Check sheet for the modelled part. Datum: model origin and axes. Units: mm. Round coordinates to 2 decimals unless told otherwise and drop trailing zeros. Write item = value, one per line.
from build123d import *

# Parameters (mm, degrees)
SKETCH1_W                                          = 308.737
SKETCH1_H                                          = 580.9742
BOSS_EXTRUDE1_STOCK_DEPTH                          = 6.35
CUT_EXTRUDE1_MOUNTING_DEPTH                        = 658.943674439
CUT_EXTRUDE1_MOUNTING_DEPTH_BACK                   = 658.943674439
SKETCH2_R                                          = 3.175
CUT_EXTRUDE2_ELEVATOR_CLEARANCE_DEPTH              = 658.943674439
CUT_EXTRUDE2_ELEVATOR_CLEARANCE_DEPTH_BACK         = 658.943674439
SKETCH3_W                                          = 66.04
SKETCH3_H                                          = 431.1142
CUT_EXTRUDE3_SCORER_ANGLE_MATERIAL_REMO_DEPTH      = 658.943674439
CUT_EXTRUDE3_SCORER_ANGLE_MATERIAL_REMO_DEPTH_BACK = 658.943674439
CUT_EXTRUDE4_ALGAE_BEARING_HOLES_DEPTH             = 658.943674439
CUT_EXTRUDE4_ALGAE_BEARING_HOLES_DEPTH_BACK        = 658.943674439
SKETCH5_R                                          = 14.224
CUT_EXTRUDE5_MOTOR_MOUNTING_HOLES_DEPTH            = 658.943674439
CUT_EXTRUDE5_MOTOR_MOUNTING_HOLES_DEPTH_BACK       = 658.943674439
SKETCH6_R                                          = 2.5527
CUT_EXTRUDE6_ALGAE_FITMENT_DEPTH                   = 658.943674439
CUT_EXTRUDE6_ALGAE_FITMENT_DEPTH_BACK              = 658.943674439
SKETCH7_R                                          = 203.2
CUT_EXTRUDE7_TOP_BOTTOM_MOUNTING_DEPTH             = 658.943674439
CUT_EXTRUDE7_TOP_BOTTOM_MOUNTING_DEPTH_BACK        = 658.943674439
SKETCH8_R                                          = 2.5527
FILLET1_R                                          = 101.6
FILLET2_R                                          = 101.6
FILLET3_R                                          = 12.7
CUT_EXTRUDE1_DEPTH                                 = 658.943674439
CUT_EXTRUDE1_DEPTH_BACK                            = 658.943674439
SKETCH9_R                                          = 3.175
CUT_EXTRUDE2_DEPTH                                 = 658.943674439
CUT_EXTRUDE2_DEPTH_BACK                            = 658.943674439
SKETCH11_R                                         = 2.5527
CUT_EXTRUDE3_DEPTH                                 = 658.943674439
CUT_EXTRUDE3_DEPTH_BACK                            = 658.943674439
SKETCH12_R                                         = 2.5527


with BuildPart() as part:
    # Sketch1 → Boss-Extrude1 _Stock (new body)
    with BuildSketch(Plane.XY):
        with Locations((154.3685, 290.4871)):
            Rectangle(SKETCH1_W, SKETCH1_H)
    extrude(amount=BOSS_EXTRUDE1_STOCK_DEPTH)

    # Sketch2 → Cut-Extrude1 _Mounting (cut, two sides: drawn at the far end of the back side and taken through both)
    with BuildSketch(Plane.XY.offset(6.35).offset(-CUT_EXTRUDE1_MOUNTING_DEPTH_BACK)):
        with Locations((12.7, 11.43)):
            Circle(SKETCH2_R)
        with Locations((12.7, 49.53)):
            Circle(SKETCH2_R)
        with Locations((12.7, 74.93)):
            Circle(SKETCH2_R)
        with Locations((12.7, 100.33)):
            Circle(SKETCH2_R)
        with Locations((12.7, 138.43)):
            Circle(SKETCH2_R)
        with Locations(Location((38.1, 11.43, 0), (0, 0, 180))):
            Circle(SKETCH2_R)
        with Locations(Location((38.1, 49.53, 0), (0, 0, 180))):
            Circle(SKETCH2_R)
        with Locations(Location((38.1, 74.93, 0), (0, 0, 180))):
            Circle(SKETCH2_R)
        with Locations(Location((38.1, 100.33, 0), (0, 0, 180))):
            Circle(SKETCH2_R)
        with Locations(Location((38.1, 138.43, 0), (0, 0, 180))):
            Circle(SKETCH2_R)
    extrude(amount=CUT_EXTRUDE1_MOUNTING_DEPTH + CUT_EXTRUDE1_MOUNTING_DEPTH_BACK, mode=Mode.SUBTRACT)

    # Sketch3 → Cut-Extrude2 _Elevator Clearance (cut, two sides: drawn at the far end of the back side and taken through both)
    with BuildSketch(Plane.XY.offset(6.35).offset(-CUT_EXTRUDE2_ELEVATOR_CLEARANCE_DEPTH_BACK)):
        with Locations((33.02, 365.4171)):
            Rectangle(SKETCH3_W, SKETCH3_H)
    extrude(amount=CUT_EXTRUDE2_ELEVATOR_CLEARANCE_DEPTH + CUT_EXTRUDE2_ELEVATOR_CLEARANCE_DEPTH_BACK, mode=Mode.SUBTRACT)

    # Sketch4 → Cut-Extrude3 _Scorer Angle Material Remo (cut, two sides: drawn at the far end of the back side and taken through both)
    with BuildSketch(Plane.XY.offset(6.35).offset(-CUT_EXTRUDE3_SCORER_ANGLE_MATERIAL_REMO_DEPTH_BACK)):
        Polygon((66.04, 580.9742), (308.737, 527.169570461), (308.737, 580.9742), align=None)
    extrude(amount=CUT_EXTRUDE3_SCORER_ANGLE_MATERIAL_REMO_DEPTH + CUT_EXTRUDE3_SCORER_ANGLE_MATERIAL_REMO_DEPTH_BACK, mode=Mode.SUBTRACT)

    # Sketch5 → Cut-Extrude4 _Algae Bearing Holes (cut, two sides: drawn at the far end of the back side and taken through both)
    with BuildSketch(Plane.XY.offset(6.35).offset(-CUT_EXTRUDE4_ALGAE_BEARING_HOLES_DEPTH_BACK)):
        with Locations((198.19747, 241.079274)):
            Circle(SKETCH5_R)
        with Locations((257.937, 314.325)):
            Circle(SKETCH5_R)
        with Locations((123.713603803, 241.079274)):
            Circle(SKETCH5_R)
    extrude(amount=CUT_EXTRUDE4_ALGAE_BEARING_HOLES_DEPTH + CUT_EXTRUDE4_ALGAE_BEARING_HOLES_DEPTH_BACK, mode=Mode.SUBTRACT)

    # Sketch6 → Cut-Extrude5 _Motor Mounting Holes (cut, two sides: drawn at the far end of the back side and taken through both)
    with BuildSketch(Plane.XY.offset(6.35).offset(-CUT_EXTRUDE5_MOTOR_MOUNTING_HOLES_DEPTH_BACK)):
        with Locations((216.157982242, 259.039786242)):
            Circle(SKETCH6_R)
        with Locations((180.236957758, 259.039786242)):
            Circle(SKETCH6_R)
        with Locations((180.236957758, 223.118761758)):
            Circle(SKETCH6_R)
        with Locations((216.157982242, 223.118761758)):
            Circle(SKETCH6_R)
        with Locations((141.674116045, 259.039786242)):
            Circle(SKETCH6_R)
        with Locations((141.674116045, 223.118761758)):
            Circle(SKETCH6_R)
        with Locations((105.753091561, 223.118761758)):
            Circle(SKETCH6_R)
        with Locations((105.753091561, 259.039786242)):
            Circle(SKETCH6_R)
    extrude(amount=CUT_EXTRUDE5_MOTOR_MOUNTING_HOLES_DEPTH + CUT_EXTRUDE5_MOTOR_MOUNTING_HOLES_DEPTH_BACK, mode=Mode.SUBTRACT)

    # Sketch7 → Cut-Extrude6 _Algae Fitment (cut, two sides: drawn at the far end of the back side and taken through both)
    with BuildSketch(Plane.XY.offset(6.35).offset(-CUT_EXTRUDE6_ALGAE_FITMENT_DEPTH_BACK)):
        with Locations((416.687, 154.686)):
            Circle(SKETCH7_R)
    extrude(amount=CUT_EXTRUDE6_ALGAE_FITMENT_DEPTH + CUT_EXTRUDE6_ALGAE_FITMENT_DEPTH_BACK, mode=Mode.SUBTRACT)

    # Sketch8 → Cut-Extrude7 _Top_Bottom Mounting (cut, two sides: drawn at the far end of the back side and taken through both)
    with BuildSketch(Plane.XY.offset(6.35).offset(-CUT_EXTRUDE7_TOP_BOTTOM_MOUNTING_DEPTH_BACK)):
        with Locations((81.187742374, 558.103501617)):
            Circle(SKETCH8_R)
        with Locations((105.985660955, 396.505737337)):
            Circle(SKETCH8_R)
        with Locations((81.187742374, 402.003303531)):
            Circle(SKETCH8_R)
        with Locations((196.937583324, 376.342181591)):
            Circle(SKETCH8_R)
        with Locations((221.735501905, 370.844615397)):
            Circle(SKETCH8_R)
        with Locations((246.533420485, 365.347049203)):
            Circle(SKETCH8_R)
        with Locations((271.331339066, 359.849483008)):
            Circle(SKETCH8_R)
        with Locations((296.129257647, 354.351916814)):
            Circle(SKETCH8_R)
        with Locations((105.985660955, 552.605935423)):
            Circle(SKETCH8_R)
        with Locations((130.783579536, 547.108369229)):
            Circle(SKETCH8_R)
        with Locations((155.581498117, 541.610803035)):
            Circle(SKETCH8_R)
        with Locations((180.379416697, 536.113236841)):
            Circle(SKETCH8_R)
        with Locations((205.177335278, 530.615670647)):
            Circle(SKETCH8_R)
        with Locations((229.975253859, 525.118104453)):
            Circle(SKETCH8_R)
        with Locations((254.77317244, 519.620538259)):
            Circle(SKETCH8_R)
        with Locations((279.571091021, 514.122972065)):
            Circle(SKETCH8_R)
    extrude(amount=CUT_EXTRUDE7_TOP_BOTTOM_MOUNTING_DEPTH + CUT_EXTRUDE7_TOP_BOTTOM_MOUNTING_DEPTH_BACK, mode=Mode.SUBTRACT)

    # Fillet1
    fillet1_edges = [part.edges().sort_by_distance(p)[0] for p in [
        (308.737, 326.840109739, 3.175),
    ]]
    fillet(fillet1_edges, radius=FILLET1_R)

    # Fillet2
    fillet2_edges = [part.edges().sort_by_distance(p)[0] for p in [
        (284.920231033, 0, 3.175),
    ]]
    fillet(fillet2_edges, radius=FILLET2_R)

    # Fillet3
    fillet3_edges = [part.edges().sort_by_distance(p)[0] for p in [
        (66.04, 149.86, 3.175),
    ]]
    fillet(fillet3_edges, radius=FILLET3_R)

    # Sketch9 → Cut-Extrude1 (cut, two sides: drawn at the far end of the back side and taken through both)
    with BuildSketch(Plane.XY.offset(6.35).offset(-CUT_EXTRUDE1_DEPTH_BACK)):
        with Locations((85.09, 162.56)):
            Circle(SKETCH9_R)
        with Locations((152.4, 19.05)):
            Circle(SKETCH9_R)
        with Locations((203.2, 76.2)):
            Circle(SKETCH9_R)
        with Locations((85.09, 378.46)):
            Circle(SKETCH9_R)
        with Locations((203.2, 190.5)):
            Circle(SKETCH9_R)
    extrude(amount=CUT_EXTRUDE1_DEPTH + CUT_EXTRUDE1_DEPTH_BACK, mode=Mode.SUBTRACT)

    # Sketch11 → Cut-Extrude2 (cut, two sides: drawn at the far end of the back side and taken through both)
    with BuildSketch(Plane.XY.offset(6.35).offset(-CUT_EXTRUDE2_DEPTH_BACK)):
        with Locations((198.197424758, 266.479274)):
            Circle(SKETCH11_R)
        with Locations((223.59747, 241.079319242)):
            Circle(SKETCH11_R)
        with Locations((172.79747, 241.079319242)):
            Circle(SKETCH11_R)
        with Locations((198.197424758, 215.679274)):
            Circle(SKETCH11_R)
    extrude(amount=CUT_EXTRUDE2_DEPTH + CUT_EXTRUDE2_DEPTH_BACK, mode=Mode.SUBTRACT)

    # Sketch12 → Cut-Extrude3 (cut, two sides: drawn at the far end of the back side and taken through both)
    with BuildSketch(Plane.XY.offset(6.35).offset(-CUT_EXTRUDE3_DEPTH_BACK)):
        with Locations((123.713558561, 266.479274)):
            Circle(SKETCH12_R)
        with Locations((149.113603803, 241.079319242)):
            Circle(SKETCH12_R)
        with Locations((123.713649045, 215.679274)):
            Circle(SKETCH12_R)
        with Locations((98.313603803, 241.079228758)):
            Circle(SKETCH12_R)
    extrude(amount=CUT_EXTRUDE3_DEPTH + CUT_EXTRUDE3_DEPTH_BACK, mode=Mode.SUBTRACT)


solid = part.part
(1) Go/stop test with flat-tipped pins: P1, Ø3, axis at x = 118.5, z = 4.5, coming from the +Y side; P2, Ø1.5, axis at y = 227.5, z = 4, coming from the +X side. Record where each tip stops, or that it passes through.
Worked answers:
P1 = 569.68
P2 = 227.27
(2) Release check for a two-part mould opening along Y. For faces 1 (the cylindrical face through (131.36, 253.073, 3.131)), 2 (the cylindrical face through (300.233, 335.336, 3.131)), 3 (the cylindrical face through (62.22, 153.48, 3.22)), 4 (the flat face through (152, 295, 6.35)) record: pulls with the +Y half, pulls with the -Y half, needs draft (parallel to the pull), parting line crosses it, or undercut.
Worked answers:
face_1 = undercut
face_2 = pulls with the -Y half
face_3 = pulls with the +Y half
face_4 = needs draft
(3) Material ranges on L1, parallel to Y at x = 38.1, z = 3 (3 decimals); L2, parallel to X at y = 254, z = 5; L3, parallel to X at y = 232.5, z = 2, recorded low to high. Write a range as [from, to].
Worked answers:
L1 = [0, 8.255], [14.605, 46.355], [52.705, 71.755], [78.105, 97.155], [103.505, 135.255], [141.605, 149.86]
L2 = [66.04, 117.77], [129.66, 192.25], [204.15, 239.41]
L3 = [66.04, 112.37], [135.06, 186.85], [209.54, 228.98]
(4) Sectioned sample at A-A on z = 1.5. Count the separate pieces of the cut face and the enclosed holes in it, then the cut area to 3 significant figures.
Worked answers:
separate_pieces = 1
enclosed_holes = 50
area = 113,000 mm²
